Can you work these out from the model? Positions are in its coordinate system, mm. Face numbers are marked on the shaded views. Round coordinates to 2 decimals unless told otherwise and drop trailing zeros. Loops run counter-clockwise (first coordinate to the right, second up) from the corner with the lowest first, then second, coordinate; pieces in that order, holes last. Notation, with made-up numbers: (2.5, 45) -> (25.5, 45) arc R7 ccw to (25.5, 50) -> close; hole circle Ø6 at (51, -6.75). An arc over 180 degrees is marked (long way). Write item = value, one per line.
from build123d import *

# Parameters (mm, degrees)
SKETCH1_W           = 205
SKETCH1_H           = 71
SKETCH1_R           = 14
SKETCH1_R_2         = 12
SKETCH1_R_3         = 1.5
BOSS_EXTRUDE1_DEPTH = 3
SKETCH2_W           = 3
SKETCH2_H           = 15
BOSS_EXTRUDE2_DEPTH = 15
BOSS_EXTRUDE3_START = -71
SKETCH2_2_W         = 3
SKETCH2_2_H         = 15
BOSS_EXTRUDE3_DEPTH = 15
SKETCH4_W           = 15
SKETCH4_H           = 3
BOSS_EXTRUDE4_DEPTH = 18
BOSS_EXTRUDE5_DEPTH = 3
CUT_EXTRUDE1_REACH  = 219.692


with BuildPart() as part:
    # Sketch1 → Boss-Extrude1 (new body)
    with BuildSketch(Plane.XY):
        with Locations((-102.5, 35.5)):
            Rectangle(SKETCH1_W, SKETCH1_H)
        with Locations((-30, 35.5)):
            Circle(SKETCH1_R, mode=Mode.SUBTRACT)
        with Locations((-80, 35.5)):
            Circle(SKETCH1_R, mode=Mode.SUBTRACT)
        with Locations((-130, 35.5)):
            Circle(SKETCH1_R, mode=Mode.SUBTRACT)
        with Locations((-177.5, 35.5)):
            Circle(SKETCH1_R_2, mode=Mode.SUBTRACT)
        with Locations((-30, 59.5)):
            Circle(SKETCH1_R_3, mode=Mode.SUBTRACT)
        with Locations((-30, 11.5)):
            Circle(SKETCH1_R_3, mode=Mode.SUBTRACT)
        with Locations((-80, 59.5)):
            Circle(SKETCH1_R_3, mode=Mode.SUBTRACT)
        with Locations((-80, 11.5)):
            Circle(SKETCH1_R_3, mode=Mode.SUBTRACT)
        with Locations((-130, 59.5)):
            Circle(SKETCH1_R_3, mode=Mode.SUBTRACT)
        with Locations((-130, 11.5)):
            Circle(SKETCH1_R_3, mode=Mode.SUBTRACT)
    extrude(amount=BOSS_EXTRUDE1_DEPTH)

    # Sketch2 → Boss-Extrude2 (add)
    with BuildSketch(Plane(origin=(0, 71, 0), x_dir=(1, 0, 0), z_dir=(0, 1, 0))):
        with Locations((-1.5, 7.5)):
            Rectangle(SKETCH2_W, SKETCH2_H)
    extrude(amount=-BOSS_EXTRUDE2_DEPTH)

    # Sketch2<2> → Boss-Extrude3 (add)
    with BuildSketch(Plane(origin=(0, 71, 0), x_dir=(1, 0, 0), z_dir=(0, 1, 0)).offset(BOSS_EXTRUDE3_START)):
        with Locations((-1.5, 7.5)):
            Rectangle(SKETCH2_2_W, SKETCH2_2_H)
    extrude(amount=BOSS_EXTRUDE3_DEPTH)

    # Sketch4 → Boss-Extrude4 (add)
    with BuildSketch(Plane.ZY.offset(205)):
        with Locations((-7.5, 1.5)):
            Rectangle(SKETCH4_W, SKETCH4_H)
    extrude(amount=-BOSS_EXTRUDE4_DEPTH)

    # Sketch5 → Boss-Extrude5 (add)
    with BuildSketch(Plane.ZY.offset(205)):
        Polygon((0, 37), (-15, 3), (0, 3), align=None)
    extrude(amount=-BOSS_EXTRUDE5_DEPTH)

    # Sketch6 → Cut-Extrude1 (cut, up to next)
    with BuildSketch(Plane.XY.offset(3), mode=Mode.PRIVATE) as cut_extrude1_sk1:
        with BuildLine():
            ThreePointArc((-182.5, 51.748076809), (-194.5, 35.5), (-182.5, 19.251923191))
            Line((-182.5, 19.251923191), (-182.5, 5))
            Line((-182.5, 5), (-200, 5))
            Line((-200, 5), (-200, 66))
            Line((-200, 66), (-182.5, 66))
            Line((-182.5, 66), (-182.5, 51.748076809))
        make_face()
    cut_extrude1_tool1 = extrude(cut_extrude1_sk1.sketch, amount=-CUT_EXTRUDE1_REACH, mode=Mode.PRIVATE) & part.part
    # Sketch6 → Cut-Extrude1 (cut, up to next)
    with BuildSketch(Plane.XY.offset(3), mode=Mode.PRIVATE) as cut_extrude1_sk2:
        with BuildLine():
            ThreePointArc((-135, 53.83030278), (-149, 35.5), (-135, 17.16969722))
            Line((-135, 17.16969722), (-135, 5))
            Line((-135, 5), (-172.5, 5))
            Line((-172.5, 5), (-172.5, 19.251923191))
            ThreePointArc((-172.5, 19.251923191), (-160.5, 35.5), (-172.5, 51.748076809))
            Line((-172.5, 51.748076809), (-172.5, 66))
            Line((-172.5, 66), (-135, 66))
            Line((-135, 66), (-135, 53.83030278))
        make_face()
    cut_extrude1_tool2 = extrude(cut_extrude1_sk2.sketch, amount=-CUT_EXTRUDE1_REACH, mode=Mode.PRIVATE) & part.part
    # Sketch6 → Cut-Extrude1 (cut, up to next)
    with BuildSketch(Plane.XY.offset(3), mode=Mode.PRIVATE) as cut_extrude1_sk3:
        with BuildLine():
            ThreePointArc((-125, 17.16969722), (-111, 35.5), (-125, 53.83030278))
            Line((-125, 53.83030278), (-125, 66))
            Line((-125, 66), (-85, 66))
            Line((-85, 66), (-85, 53.83030278))
            ThreePointArc((-85, 53.83030278), (-99, 35.5), (-85, 17.16969722))
            Line((-85, 17.16969722), (-85, 5))
            Line((-85, 5), (-125, 5))
            Line((-125, 5), (-125, 17.16969722))
        make_face()
    cut_extrude1_tool3 = extrude(cut_extrude1_sk3.sketch, amount=-CUT_EXTRUDE1_REACH, mode=Mode.PRIVATE) & part.part
    # Sketch6 → Cut-Extrude1 (cut, up to next)
    with BuildSketch(Plane.XY.offset(3), mode=Mode.PRIVATE) as cut_extrude1_sk4:
        with BuildLine():
            ThreePointArc((-75, 17.16969722), (-61, 35.5), (-75, 53.83030278))
            Line((-75, 53.83030278), (-75, 66))
            Line((-75, 66), (-35, 66))
            Line((-35, 66), (-35, 53.83030278))
            ThreePointArc((-35, 53.83030278), (-49, 35.5), (-35, 17.16969722))
            Line((-35, 17.16969722), (-35, 5))
            Line((-35, 5), (-75, 5))
            Line((-75, 5), (-75, 17.16969722))
        make_face()
    cut_extrude1_tool4 = extrude(cut_extrude1_sk4.sketch, amount=-CUT_EXTRUDE1_REACH, mode=Mode.PRIVATE) & part.part
    # Sketch6 → Cut-Extrude1 (cut, up to next)
    with BuildSketch(Plane.XY.offset(3), mode=Mode.PRIVATE) as cut_extrude1_sk5:
        with BuildLine():
            ThreePointArc((-25, 17.16969722), (-11, 35.5), (-25, 53.83030278))
            Line((-25, 53.83030278), (-25, 66))
            Line((-25, 66), (-5, 66))
            Line((-5, 66), (-5, 5))
            Line((-5, 5), (-25, 5))
            Line((-25, 5), (-25, 17.16969722))
        make_face()
    cut_extrude1_tool5 = extrude(cut_extrude1_sk5.sketch, amount=-CUT_EXTRUDE1_REACH, mode=Mode.PRIVATE) & part.part
    add(cut_extrude1_tool1.solids().sort_by_distance((-195.134606, 35.5, 3))[0], mode=Mode.SUBTRACT)
    add(cut_extrude1_tool2.solids().sort_by_distance((-154.340944, 35.5, 3))[0], mode=Mode.SUBTRACT)
    add(cut_extrude1_tool3.solids().sort_by_distance((-105, 35.5, 3))[0], mode=Mode.SUBTRACT)
    add(cut_extrude1_tool4.solids().sort_by_distance((-55, 35.5, 3))[0], mode=Mode.SUBTRACT)
    add(cut_extrude1_tool5.solids().sort_by_distance((-10.35805, 35.5, 3))[0], mode=Mode.SUBTRACT)


solid = part.part
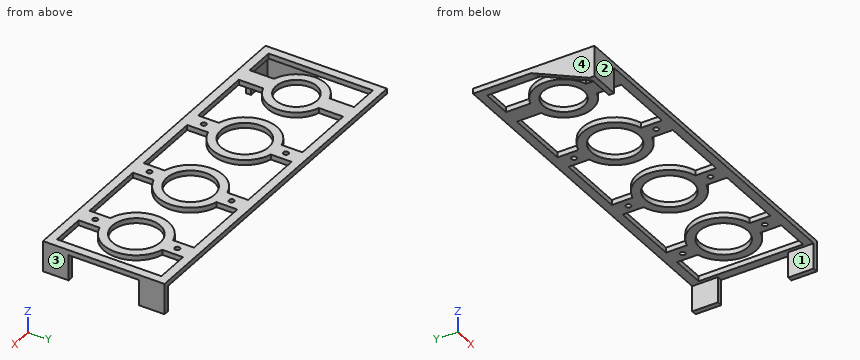
1. Suppose I cut it at C-C, the plane y = 7.5. List the corners of the cut face in (x, z) for me.
Entries:
outline = (-205, -13.01) -> (-202, -13.01) -> (-202, 0) -> (-200, 0) -> (-200, 3) -> (-205, 3) -> close; (-182.5, 0) -> (-172.5, 0) -> (-172.5, 3) -> (-182.5, 3) -> close; (-135, 0) -> (-125, 0) -> (-125, 3) -> (-135, 3) -> close; (-85, 0) -> (-75, 0) -> (-75, 3) -> (-85, 3) -> close; (-35, 0) -> (-25, 0) -> (-25, 3) -> (-35, 3) -> close; (-5, 0) -> (-3, 0) -> (-3, -15) -> (0, -15) -> (0, 3) -> (-5, 3) -> close
2. Suppose I cut it at B-B, the plane x = -177.5. List the corners of the cut face in (y, z) for me.
Entries:
outline = (0, 0) -> (23.5, 0) -> (23.5, 3) -> (0, 3) -> close; (47.5, 0) -> (71, 0) -> (71, 3) -> (47.5, 3) -> close
3. I need wall thicknesses on line 1 (Y direction, x = -151, z = 0.5); line 2 (Z direction, x = -63, y = 4.5); line 3 (Y direction, x = -37.5, z = 1.75). Which ranges of each line are inside material? Lowest first, please. Write a range as [from, to].
Entries:
line_1 = [0, 5], [66, 71]
line_2 = [0, 3]
line_3 = [0, 5], [18.04, 23.68], [47.32, 52.96], [66, 71]
4. Suppose I cut it at A-A, the plane z = -10.5. List the corners of the cut face in (x, y) for me.
Entries:
outline = (-205, 0) -> (-187, 0) -> (-187, 3) -> (-202, 3) -> (-202, 13.2) -> (-205, 13.2) -> close; (-3, 0) -> (0, 0) -> (0, 15) -> (-3, 15) -> close; (-3, 56) -> (0, 56) -> (0, 71) -> (-3, 71) -> close
5. We'd pull the mould along X, two halves only. Please class the marked faces 1, 2, 3 and 4: released by +X, released by -X, zero draft, split by the parting line, or undercut.
Entries:
face_1 = undercut
face_2 = zero draft
face_3 = released by +X
face_4 = released by -X
